Could you check a few things on this model? Use its own coordinates, in mm. A direction names the side the tool comes from. Give positions to 0.01 mm unless a question says otherwise; leave off trailing zeros. Order: outer loops, then holes, each group sorted by start corner. A loop starts at its lowest first (then second) coordinate and runs counter-clockwise, first axis right, second up. Notation, with made-up numbers: M -39.75,16 L -32.75,16 A8 ccw -32.75,25 Z; hole C -17,12.25 d3. An arc over 180 degrees is marked long. Use a Markdown table: item, result. Add a question column.
Item 1: Suppose I cut it at D-D on y = 9. Write out the boundary of the cut face in (x, z), plus the area to 3 significant figures.
Item 2: Suppose I cut it at C-C on y = 1.75. Write out the boundary of the cut face in (x, z).
Item 3: For faces 4 (the face through (-4.6, 3, 7)), 5 (the face through (-6.52, 23.72, 0.99)), 6 (the face through (0, 5, 7)), which set-ups out of +Z, -Z, +X, -X, +Y, -Y let a thin tool reach every point of the face, with its end or its side?
Item 4: I'm going to push flat-ended pins straight in: pin 1 Ø1.5 at (y, z) = (2.5, 6) entering from +X; pin 2 Ø2 at (y, z) = (11.5, 3.5) entering from -X; pin 3 Ø4 at (y, z) = (3.5, 6) entering from -X; pin 4 Ø3.5 at (x, z) = (0, 8.8) entering from +Y. Where does each tip first touch, or does it pass through?
Item 5: Suppose I cut it at A-A on x = 0. Write out the boundary of the cut face in (y, z), plus the area to 3 significant figures.
Item 6: If I drill on L1, parallel to Z at x = -1.5, y = 7.5; L2, parallel to Y at x = 1.75, z = 10; L3, parallel to Z at x = 4.25, y = 3.5, over which ranges is the centre line in solid material (lowest first)? Write a range as from..to.
Item 7: If we mould it in two halves opening along X, with no side actions, what happens to faces 1 (the face through (4.6, 3, 7)), 2 (the face through (6.88, 24.02, 0.99)), 3 (the face through (0, 0, 5))? For each: released by +X, released by -X, zero draft, split by the parting line, or undercut.
Item 8: Suppose I cut it at B-B on z = 8.8. Write out the boundary of the cut face in (x, y), plus the area to 3 significant figures.
from build123d import *

# Parameters (mm, degrees)
SKETCH1_W           = 27
SKETCH1_H           = 26
BOSS_EXTRUDE1_DEPTH = 2
SKETCH2_W           = 27
SKETCH2_H           = 5
BOSS_EXTRUDE2_DEPTH = 10
CUT_EXTRUDE1_REACH  = 28
SKETCH3_R           = 1.6
SKETCH4_W           = 8.9
SKETCH4_H           = 10
CUT_EXTRUDE2_DEPTH  = 5
CUT_EXTRUDE3_REACH  = 14
SKETCH5_R           = 1.8
FILLET1_R           = 5
FILLET2_R           = 2
FILLET3_R           = 2


with BuildPart() as part:
    # Sketch1 → Boss-Extrude1 (new body)
    with BuildSketch(Plane.XY):
        with Locations((0, 13)):
            Rectangle(SKETCH1_W, SKETCH1_H)
    extrude(amount=BOSS_EXTRUDE1_DEPTH)

    # Sketch2 → Boss-Extrude2 (add)
    with BuildSketch(Plane.XY.offset(2)):
        with Locations((0, 2.5)):
            Rectangle(SKETCH2_W, SKETCH2_H)
    extrude(amount=BOSS_EXTRUDE2_DEPTH)

    # Sketch3 → Cut-Extrude1 (cut, up to next)
    with BuildSketch(Plane.XZ, mode=Mode.PRIVATE) as cut_extrude1_sk1:
        with Locations((0, 8.8)):
            Circle(SKETCH3_R)
    cut_extrude1_tool1 = extrude(cut_extrude1_sk1.sketch, amount=-CUT_EXTRUDE1_REACH, mode=Mode.PRIVATE) & part.part
    add(cut_extrude1_tool1.solids().sort_by_distance((0, 0, 8.8))[0], mode=Mode.SUBTRACT)

    # Sketch4 → Cut-Extrude2 (cut)
    with BuildSketch(Plane(origin=(0, 5, 0), x_dir=(1, 0, 0), z_dir=(0, 1, 0))):
        with Locations((9.05, -7)):
            Rectangle(SKETCH4_W, SKETCH4_H)
    cut_extrude2 = extrude(amount=-CUT_EXTRUDE2_DEPTH, mode=Mode.SUBTRACT)

    # Mirror1: Cut-Extrude2 across plane
    add(cut_extrude2.mirror(Plane(origin=(0, 0, 0), x_dir=(0, 0, 1), z_dir=(1, 0, 0))), mode=Mode.SUBTRACT)

    # Sketch5 → Cut-Extrude3 (cut, up to next)
    with BuildSketch(Plane(origin=(0, 0, 0), x_dir=(-1, 0, 0), z_dir=(0, 0, -1)), mode=Mode.PRIVATE) as cut_extrude3_sk1:
        with Locations((-7.845874534, 22.5)):
            Circle(SKETCH5_R)
    cut_extrude3_tool1 = extrude(cut_extrude3_sk1.sketch, amount=-CUT_EXTRUDE3_REACH, mode=Mode.PRIVATE) & part.part
    add(cut_extrude3_tool1.solids().sort_by_distance((7.845875, 22.5, 0))[0], mode=Mode.SUBTRACT)
    # Sketch5 → Cut-Extrude3 (cut, up to next)
    with BuildSketch(Plane(origin=(0, 0, 0), x_dir=(-1, 0, 0), z_dir=(0, 0, -1)), mode=Mode.PRIVATE) as cut_extrude3_sk2:
        with Locations((7.845874534, 22.5)):
            Circle(SKETCH5_R)
    cut_extrude3_tool2 = extrude(cut_extrude3_sk2.sketch, amount=-CUT_EXTRUDE3_REACH, mode=Mode.PRIVATE) & part.part
    add(cut_extrude3_tool2.solids().sort_by_distance((-7.845875, 22.5, 0))[0], mode=Mode.SUBTRACT)
    # Sketch5 → Cut-Extrude3 (cut, up to next)
    with BuildSketch(Plane(origin=(0, 0, 0), x_dir=(-1, 0, 0), z_dir=(0, 0, -1)), mode=Mode.PRIVATE) as cut_extrude3_sk3:
        with Locations((-9.846580197, 9)):
            Circle(SKETCH5_R)
    cut_extrude3_tool3 = extrude(cut_extrude3_sk3.sketch, amount=-CUT_EXTRUDE3_REACH, mode=Mode.PRIVATE) & part.part
    add(cut_extrude3_tool3.solids().sort_by_distance((9.84658, 9, 0))[0], mode=Mode.SUBTRACT)
    # Sketch5 → Cut-Extrude3 (cut, up to next)
    with BuildSketch(Plane(origin=(0, 0, 0), x_dir=(-1, 0, 0), z_dir=(0, 0, -1)), mode=Mode.PRIVATE) as cut_extrude3_sk4:
        with Locations((9.846580197, 9)):
            Circle(SKETCH5_R)
    cut_extrude3_tool4 = extrude(cut_extrude3_sk4.sketch, amount=-CUT_EXTRUDE3_REACH, mode=Mode.PRIVATE) & part.part
    add(cut_extrude3_tool4.solids().sort_by_distance((-9.84658, 9, 0))[0], mode=Mode.SUBTRACT)

    # Fillet1
    fillet1_edges = [part.edges().sort_by_distance(p)[0] for p in [
        (-13.5, 26, 1),
        (13.5, 26, 1),
    ]]
    fillet(fillet1_edges, radius=FILLET1_R)

    # Fillet2
    fillet2_edges = [part.edges().sort_by_distance(p)[0] for p in [
        (0, 5, 2),
        (4.6, 2.5, 2),
        (-4.6, 2.5, 2),
    ]]
    fillet(fillet2_edges, radius=FILLET2_R)

    # Fillet3
    fillet3_edges = [part.edges().sort_by_distance(p)[0] for p in [
        (4.6, 2.5, 12),
        (-4.6, 2.5, 12),
    ]]
    fillet(fillet3_edges, radius=FILLET3_R)


solid = part.part
Findings below:
| question | item | result |
|---|---|---|
| 1 | outline | M -13.5,0 L -11.65,0 L -11.65,2 L -13.5,2 Z; M -8.05,0 L 8.05,0 L 8.05,2 L -8.05,2 Z; M 11.65,0 L 13.5,0 L 13.5,2 L 11.65,2 Z |
| 1 | area | 39.6 mm^2 |
| 2 | outline | M -13.5,0 L 13.5,0 L 13.5,2 L 6.6,2 A2 cw 4.6,4 L 4.6,10 A2 ccw 2.6,12 L -2.6,12 A2 ccw -4.6,10 L -4.6,4 A2 cw -6.6,2 L -13.5,2 Z; hole C 0,8.8 d3.2 |
| 3 | face 4 | +Z, -X, +Y, -Y |
| 3 | face 5 | +Z, -Z |
| 3 | face 6 | +Z, +X, -X, +Y |
| 4 | pin 1 | stops at x = 4.6 |
| 4 | pin 2 | passes through |
| 4 | pin 3 | stops at x = -4.6 |
| 4 | pin 4 | stops at y = 5 |
| 5 | outline | M 0,0 L 26,0 L 26,2 L 7,2 A2 cw 5,4 L 5,7.2 L 0,7.2 Z; M 0,10.4 L 5,10.4 L 5,12 L 0,12 Z |
| 5 | area | 86.9 mm^2 |
| 6 | L1 | z = 0..2 |
| 6 | L2 | y = 0..5 |
| 6 | L3 | z = 0..11.13 |
| 7 | face 1 | released by +X |
| 7 | face 2 | undercut |
| 7 | face 3 | zero draft |
| 8 | outline | M -4.6,0 L -1.6,0 L -1.6,5 L -4.6,5 Z; M 1.6,0 L 4.6,0 L 4.6,5 L 1.6,5 Z |
| 8 | area | 30.0 mm^2 |
